Geometry check sheet. Reference: the model listing, model coordinates, mm. A direction names the side the tool comes from. Give positions to 0.01 mm unless a question says otherwise; leave off trailing zeros. Write each loop counter-clockwise with the first axis right and the second up, starting at its lowest first coordinate (ties: lowest second). Pieces come first, ordered by that corner, then holes. Notation, with made-up numbers: (3.5, 40.5) -> (29.5, 40.5) arc R22 ccw to (29.5, 49.5) -> close; hole circle Ø9 at (78, 36). An arc over 180 degrees is marked (long way). One line per item, written item: value.
from build123d import *

# Parameters (mm, degrees)
SKETCH_1_W          = 190
SKETCH_1_H          = 140
EXTRUDE_1_DEPTH     = 10
FILLET_1_R          = 5
SKETCH_2_R          = 32.5
EXTRUDE_2_DEPTH     = 20
SKETCH_3_R          = 20
EXTRUDE_3_DEPTH     = 10
SKETCH_4_R          = 10
EXTRUDE_4_DEPTH     = 20
CUT_EXTRUDE_START   = -10
SKETCH_5_R          = 10
SKETCH_5_R_2        = 4
CUT_EXTRUDE_1_DEPTH = 10
SKETCH_6_R          = 10
SKETCH_6_R_2        = 4
CUT_EXTRUDE_2_DEPTH = 10
SKETCH_7_R          = 4
EXTRUDE_5_DEPTH     = 10
SKETCH_8_R          = 2.5
CUT_EXTRUDE_3_DEPTH = 10


with BuildPart() as part:
    # 草图1 → 凸台-拉伸1 (new body)
    with BuildSketch(Plane.XY):
        Rectangle(SKETCH_1_W, SKETCH_1_H)
    extrude(amount=EXTRUDE_1_DEPTH)

    # 圆角1
    fillet_1_edges = [part.edges().sort_by_distance(p)[0] for p in [
        (-95, -70, 5),
        (-95, 70, 5),
        (95, 70, 5),
        (95, -70, 5),
    ]]
    fillet(fillet_1_edges, radius=FILLET_1_R)

    # 草图2 → 凸台-拉伸2 (add)
    with BuildSketch(Plane.XY.offset(10)):
        Circle(SKETCH_2_R)
    extrude(amount=EXTRUDE_2_DEPTH)

    # 草图3 → 凸台-拉伸3 (add)
    with BuildSketch(Plane.XY.offset(30)):
        Circle(SKETCH_3_R)
    extrude(amount=EXTRUDE_3_DEPTH)

    # 草图4 → 凸台-拉伸4 (add)
    with BuildSketch(Plane.XY.offset(40)):
        Circle(SKETCH_4_R)
    extrude(amount=EXTRUDE_4_DEPTH)

    # 草图5 → 切除-拉伸1 (cut)
    with BuildSketch(Plane.XY.offset(60).offset(CUT_EXTRUDE_START)):
        Circle(SKETCH_5_R)
        Circle(SKETCH_5_R_2, mode=Mode.SUBTRACT)
    extrude(amount=CUT_EXTRUDE_1_DEPTH, mode=Mode.SUBTRACT)

    # 草图6 → 切除-拉伸2 (cut)
    with BuildSketch(Plane.XY.offset(50).offset(CUT_EXTRUDE_START)):
        Circle(SKETCH_6_R)
        Circle(SKETCH_6_R_2, mode=Mode.SUBTRACT)
    extrude(amount=CUT_EXTRUDE_2_DEPTH, mode=Mode.SUBTRACT)

    # 草图7 → 凸台-拉伸5 (add)
    with BuildSketch(Plane.XY.offset(60)):
        Circle(SKETCH_7_R)
    extrude(amount=EXTRUDE_5_DEPTH)

    # 草图8 → 切除-拉伸3 (cut)
    with BuildSketch(Plane.XY.offset(10)):
        with Locations((82.5, 57.5)):
            Circle(SKETCH_8_R)
        with Locations(Location((82.5, -57.5, 0), (0, 0, 180))):
            Circle(SKETCH_8_R)
        with Locations((-82.5, -57.5)):
            Circle(SKETCH_8_R)
        with Locations(Location((-82.5, 57.5, 0), (0, 0, 180))):
            Circle(SKETCH_8_R)
    extrude(amount=-CUT_EXTRUDE_3_DEPTH, mode=Mode.SUBTRACT)


solid = part.part
1) Sectioned sample at C-C on x = 0. Record the cut outline in (y, z), plus the area to 3 significant figures.
Verdict:
outline: (-70, 0) -> (70, 0) -> (70, 10) -> (32.5, 10) -> (32.5, 30) -> (20, 30) -> (20, 40) -> (4, 40) -> (4, 70) -> (-4, 70) -> (-4, 40) -> (-20, 40) -> (-20, 30) -> (-32.5, 30) -> (-32.5, 10) -> (-70, 10) -> close
area: 3,340 mm^2
2) Sectioned sample at D-D on y = 0. Record the cut outline in (x, z).
Verdict:
outline: (-95, 0) -> (95, 0) -> (95, 10) -> (32.5, 10) -> (32.5, 30) -> (20, 30) -> (20, 40) -> (4, 40) -> (4, 70) -> (-4, 70) -> (-4, 40) -> (-20, 40) -> (-20, 30) -> (-32.5, 30) -> (-32.5, 10) -> (-95, 10) -> close
3) Mould release check, pull along X, two halves, no side actions. Record for faces 1 (the cylindrical face through (-0.867, -3.905, 54.79)), 2 (the cylindrical face through (-84.34, -55.81, 5.07)), 3 (the flat face through (14, 15, 30)): released by +X, released by -X, zero draft, split by the parting line, or undercut.
Verdict:
face 1: split by the parting line
face 2: undercut
face 3: zero draft
4) Tool access check on faces 4 (the cylindrical face through (-80.66, 55.81, 5.07)), 5 (the cylindrical face through (31, 9.76, 19.86)). Record the directions out of +Z, -Z, +X, -X, +Y, -Y that give a thin tool (end or side, any length) a straight path to the whole face; none if there is none.
Verdict:
face 4: +Z, -Z
face 5: +Z
5) Scan lines: probe 1 along Y at (x, z) = (-82, 5); probe 2 along Y at (x, z) = (-82.5, 6); probe 3 along X at (y, z) = (57, 6). Record each from-to range of solid material in increasing order.
Verdict:
probe 1: -70 to -59.95, -55.05 to 55.05, 59.95 to 70
probe 2: -70 to -60, -55 to 55, 60 to 70
probe 3: -95 to -84.95, -80.05 to 80.05, 84.95 to 95
6) Depth check by flat-ended pin: pin 1 Ø19.5 at (x, y) = (7.5, 9) entering from +Z; pin 2 Ø10 at (y, z) = (4.5, 41.5) entering from -X; pin 3 Ø6 at (y, z) = (6, 27.5) entering from -X; pin 4 Ø6.5 at (x, y) = (82.5, 57.5) entering from +Z. Enter the tip coordinate at first touch or a pass-through.
Verdict:
pin 1: z = 70
pin 2: x = -20
pin 3: x = -32.36
pin 4: z = 10
7) Sectioned sample at A-A on y = -57.5. Record the cut outline in (x, z), plus the area to 3 significant figures.
Verdict:
outline: (-95, 0) -> (-85, 0) -> (-85, 10) -> (-95, 10) -> close; (-80, 0) -> (80, 0) -> (80, 10) -> (-80, 10) -> close; (85, 0) -> (95, 0) -> (95, 10) -> (85, 10) -> close
area: 1,800 mm^2
8) Sectioned sample at B-B on x = 82.5. Record the cut outline in (y, z).
Verdict:
outline: (-70, 0) -> (-60, 0) -> (-60, 10) -> (-70, 10) -> close; (-55, 0) -> (55, 0) -> (55, 10) -> (-55, 10) -> close; (60, 0) -> (70, 0) -> (70, 10) -> (60, 10) -> close
